CAD build for the part. Positions are in the model's coordinates, mm. Face numbers are marked on the shaded views. A direction names the side the tool comes from. Coordinates: 2 decimals unless noted, no trailing zeros. Order: outer loops, then holes, each group sorted by start corner. A loop starts at its lowest first (then second) coordinate and runs counter-clockwise, first axis right, second up. Notation, with made-up numbers: (59.25, -6) -> (111.25, -6) arc R23 cw to (111.25, 11) -> close; hole circle Ø11 at (19, -33). An arc over 180 degrees is marked (long way). Use one line per item in the form item = value. Start each with the question number.
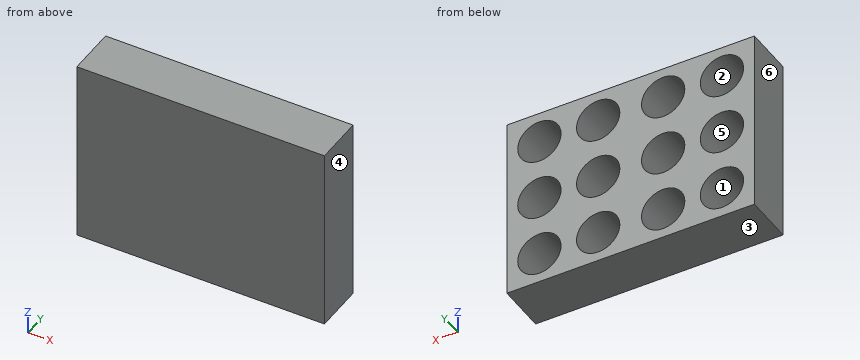
from build123d import *

# Parameters (mm, degrees)
CROQUIS1_W              = 400
CROQUIS1_H              = 300
SALIENTE_EXTRUIR1_DEPTH = 80
CROQUIS3_R              = 35
CORTAR_EXTRUIR1_DEPTH   = 70


with BuildPart() as part:
    # Croquis1 → Saliente-Extruir1 (new body)
    with BuildSketch(Plane(origin=(0, 0, 0), x_dir=(1, 0, 0), z_dir=(0, 1, 0))):
        Rectangle(CROQUIS1_W, CROQUIS1_H)
    extrude(amount=SALIENTE_EXTRUIR1_DEPTH)

    # Croquis3 → Cortar-Extruir1 (cut)
    with BuildSketch(Plane(origin=(0, 80, 0), x_dir=(1, 0, 0), z_dir=(0, 1, 0))):
        with Locations(Location((-147.5, 100, 0), (0, 0, 270))):
            Circle(CROQUIS3_R)
        with Locations(Location((-52.5, 100, 0), (0, 0, 270))):
            Circle(CROQUIS3_R)
        with Locations(Location((-147.5, 0, 0), (0, 0, 270))):
            Circle(CROQUIS3_R)
        with Locations(Location((-52.5, 0, 0), (0, 0, 270))):
            Circle(CROQUIS3_R)
        with Locations(Location((52.5, 0, 0), (0, 0, 90))):
            Circle(CROQUIS3_R)
        with Locations(Location((52.5, 100, 0), (0, 0, 90))):
            Circle(CROQUIS3_R)
        with Locations(Location((147.5, 0, 0), (0, 0, 90))):
            Circle(CROQUIS3_R)
        with Locations(Location((147.5, 100, 0), (0, 0, 90))):
            Circle(CROQUIS3_R)
        with Locations(Location((-52.5, -100, 0), (0, 0, 90))):
            Circle(CROQUIS3_R)
        with Locations(Location((-147.5, -100, 0), (0, 0, 90))):
            Circle(CROQUIS3_R)
        with Locations(Location((147.5, -100, 0), (0, 0, 270))):
            Circle(CROQUIS3_R)
        with Locations(Location((52.5, -100, 0), (0, 0, 270))):
            Circle(CROQUIS3_R)
    extrude(amount=-CORTAR_EXTRUIR1_DEPTH, mode=Mode.SUBTRACT)


solid = part.part
1) Probe L1, parallel to X at y = 42, z = 0; L2, parallel to Z at x = 52, y = 46; L3, parallel to Z at x = -123, y = 53 (3 decimals). List the from-to ranges inside material, lowest first.
2) 3-axis set-ups, long thin cutter, end or side, ignore diameter. For the marked faces 5 and 6: which of +Z, -Z, +X, -X, +Y, -Y reach the whole face in a straight line?
3) Cut at C-C on x = 147.5. Give the cut face in (y, z), then the cut area to 3 significant figures.
4) Cut at A-A on y = 59. Count the separate pieces of the cut face and the enclosed holes in it, then the cut area to 3 significant figures.
5) Drop flat-ended pins along their axis: P1, Ø21, axis at x = 48, z = 114, coming from the +Y side; P2, Ø5, axis at x = 157.5, z = 91.5, coming from the -Y side. Give the stop position or say it passes through.
6) Cut at B-B on z = -100. Give the cut face in (x, y).
7) Two-plate mould, pull along Z, no slides. Class the marked faces 1, 2, 3 and 4: released by +Z, released by -Z, zero draft, split by the parting line, or undercut.
8) Cut at D-D on x = 42. Give the cut face in (y, z).
Values follow:
q1.L1 = -200 to -182.5, -112.5 to -87.5, -17.5 to 17.5, 87.5 to 112.5, 182.5 to 200
q1.L2 = -150 to -135, -65 to -35, 35 to 65, 135 to 150
q1.L3 = -150 to -124.995, -75.005 to -24.995, 24.995 to 75.005, 124.995 to 150
q2.face_5 = +Y
q2.face_6 = +Z, -Z, -X, +Y, -Y
q3.outline = (0, -150) -> (80, -150) -> (80, -135) -> (10, -135) -> (10, -65) -> (80, -65) -> (80, -35) -> (10, -35) -> (10, 35) -> (80, 35) -> (80, 65) -> (10, 65) -> (10, 135) -> (80, 135) -> (80, 150) -> (0, 150) -> close
q3.area = 9,300 mm^2
q4.separate_pieces = 1
q4.enclosed_holes = 12
q4.area = 73,800 mm^2
q5.P1 = 10
q5.P2 = 0
q6.outline = (-200, 0) -> (200, 0) -> (200, 80) -> (182.5, 80) -> (182.5, 10) -> (112.5, 10) -> (112.5, 80) -> (87.5, 80) -> (87.5, 10) -> (17.5, 10) -> (17.5, 80) -> (-17.5, 80) -> (-17.5, 10) -> (-87.5, 10) -> (-87.5, 80) -> (-112.5, 80) -> (-112.5, 10) -> (-182.5, 10) -> (-182.5, 80) -> (-200, 80) -> close
q7.face_1 = undercut
q7.face_2 = undercut
q7.face_3 = released by -Z
q7.face_4 = zero draft
q8.outline = (0, -150) -> (80, -150) -> (80, -133.39) -> (10, -133.39) -> (10, -66.61) -> (80, -66.61) -> (80, -33.39) -> (10, -33.39) -> (10, 33.39) -> (80, 33.39) -> (80, 66.61) -> (10, 66.61) -> (10, 133.39) -> (80, 133.39) -> (80, 150) -> (0, 150) -> close
